Autodesk Inventor part; units mm, degrees
ref_plane "YZ Plane" through (0, 0, 0) normal (1, 0, 0) x (0, 1, 0)
ref_plane "XZ Plane" through (0, 0, 0) normal (0, 1, 0) x (-1, 0, 0)
ref_plane "XY Plane" through (0, 0, 0) normal (0, 0, 1) x (1, 0, 0)
sketch "Sketch1" plane through (0, 0, 0) normal (0, 1, 0) x (-1, 0, 0)
  line L0 (0, 0) -> (-13.33, 0) construction
  line L1 (0, -2.665) -> (-13.33, -2.665)
  line L2 (-13.33, 2.665) -> (0, 2.665)
  arc A0 (0, -2.665) -> (0, 2.665) centre (0, 0) ccw
  arc A1 (-13.33, 2.665) -> (-13.33, -2.665) centre (-13.33, 0) ccw
  circle A2 centre (-13.33, 0) radius 0.83
  circle A3 centre (0, 0) radius 1.33
  point P0 (-6.665, 0)
  dimension "d0" = 5.33
  dimension "d1" = 13.33
  dimension "d2" = 2.66
  dimension "d3" = 1.66
extrude "Extrusion1" add sketch "Sketch1" along normal blind 3.33
fillet "Fillet1" radius 0.33 8 edges at (6.665, 0, -2.665) (6.665, 3.33, -2.665) (-2.665, 0, 0) (6.665, 0, 2.665) (15.995, 0, 0) (-2.665, 3.33, 0) (6.665, 3.33, 2.665) (15.995, 3.33, 0)
properties part number "G-5"
Part model, mm, in its own coordinate system. Give positions to 0.01 mm unless a question says otherwise; leave off trailing zeros. Loops run counter-clockwise (first coordinate to the right, second up) from the corner with the lowest first, then second, coordinate; pieces in that order, holes last. Notation, with made-up numbers: (48.5, 54) -> (84.5, 54) arc R19 ccw to (84.5, 77) -> close; hole circle Ø9 at (-14, -6). An arc over 180 degrees is marked (long way). Write each question's results on one line, items separated by ' | '. Start each with the question number.
Q1. Band-saw the part on B-B on y = 1.6. List the corners of the cut face in (x, z) (3 decimals), plus the area to 3 significant figures.
Q2. Band-saw the part on A-A on z = 0. List the corners of the cut face in (x, y) (3 decimals).
Q3. Wall check: L1, parallel to Z at x = 0, y = 1.5 (3 decimals); L2, parallel to Z at x = 13.33, y = 1.7 (3 decimals); L3, parallel to X at y = 1.25, z = -0.2. Give the ranges that are in metal, low to high.
Q4. Band-saw the part on C-C on x = 1. List the corners of the cut face in (y, z) (3 decimals).
Q5. Pin check, flat tips, straight feed: P1, Ø1.9, axis at x = 13.33, z = 0, coming from the +Y side; P2, Ø2, axis at x = 0, z = 0, coming from the -Y side. Stop position of each tip, or through.
Q6. Pull direction X, two halves, no side cores. Call faces 1 (the face through (7, 2, -2.665)), 2 (the face through (-1.27, 1.64, -0.4)), 3 (the face through (-2.664, 1.646, 0.059)), 4 (the face through (14.16, 1.64, -0.04)): +X half, -X half, draft (parallel to the pull), parting line (faces both ways), or undercut.
Results are:
1) outline: (0, -2.665) -> (13.33, -2.665) arc R2.665 ccw to (13.33, 2.665) -> (0, 2.665) arc R2.665 ccw to start; hole circle Ø2.66 at (0, 0); hole circle Ø1.66 at (13.33, 0) | area: 85.6 mm²
2) outline: (-2.665, 0.33) arc R0.33 ccw to (-2.335, 0) -> (-1.33, 0) -> (-1.33, 3.33) -> (-2.335, 3.33) arc R0.33 ccw to (-2.665, 3) -> close; (1.33, 0) -> (12.5, 0) -> (12.5, 3.33) -> (1.33, 3.33) -> close; (14.16, 0) -> (15.665, 0) arc R0.33 ccw to (15.995, 0.33) -> (15.995, 3) arc R0.33 ccw to (15.665, 3.33) -> (14.16, 3.33) -> close
3) L1: z = -2.665 to -1.33, 1.33 to 2.665 | L2: z = -2.665 to -0.83, 0.83 to 2.665 | L3: x = -2.66 to -1.31, 1.31 to 12.52, 14.14 to 15.99
4) outline: (0, -2.335) arc R0.33 ccw to (0.33, -2.665) -> (3, -2.665) arc R0.33 ccw to (3.33, -2.335) -> (3.33, -0.877) -> (0, -0.877) -> close; (0, 0.877) -> (3.33, 0.877) -> (3.33, 2.335) arc R0.33 ccw to (3, 2.665) -> (0.33, 2.665) arc R0.33 ccw to (0, 2.335) -> close
5) P1: stops at y = 3.33 | P2: passes through
6) face 1: draft | face 2: undercut | face 3: -X half | face 4: undercut
